Build history of the part. All positions in model axes, mm. A direction names the side the tool comes from. Round coordinates to 2 decimals unless told otherwise and drop trailing zeros. Write each loop counter-clockwise with the first axis right and the second up, starting at its lowest first coordinate (ties: lowest second). Pieces come first, ordered by that corner, then holes.
Item 1: Band-saw the part on A-A, the plane x = 0. Write the cut outline in (y, z).
Item 2: Wall check: probe 1 along X at (y, z) = (-1, 0); probe 2 along Z at (x, y) = (0, 2.1). Give the ranges that are in metal, low to high.
Item 3: Band-saw the part on D-D, the plane z = 2.25. Write the cut outline in (x, y), then the cut area to 3 significant figures.
Item 4: Drop a flat-ended pin along its axis: pin 1 Ø1 at (x, y) = (-2, -0.5) entering from -Z. Give the stop position or say it passes through.
Item 5: 3-axis set-ups, long thin cutter, end or side, ignore diameter. For faces 1 (the cylindrical face through (-6, -1, 0)), 2 (the cylindrical face through (3.233, 1.479, 1.341)): which of +Z, -Z, +X, -X, +Y, -Y reach the whole face in a straight line?
Item 6: Band-saw the part on C-C, the plane y = 2.1. Write the cut outline in (x, z).
Item 7: Band-saw the part on B-B, the plane z = 0.5. Write the cut outline in (x, y), then the cut area to 3 significant figures.
```python
from build123d import *

# Parameters (mm, degrees)
SKETCH_1_R      = 3.5
SKETCH_1_R_2    = 2
EXTRUDE_1_DEPTH = 3
SKETCH_1_3_R    = 6
SKETCH_1_3_R_2  = 3.5
SKETCH_1_3_R_3  = 2
EXTRUDE_2_DEPTH = 2


with BuildPart() as part:
    # Sketch 1 → Extrude 1 (new body)
    with BuildSketch(Plane(origin=(0, 0, 0), x_dir=(1, 0, 0), z_dir=(0, 1, 0))):
        Circle(SKETCH_1_R)
        Circle(SKETCH_1_R_2, mode=Mode.SUBTRACT)
    extrude(amount=EXTRUDE_1_DEPTH)

    # Sketch 1_3 → Extrude 2 (add)
    with BuildSketch(Plane(origin=(0, 0, 0), x_dir=(1, 0, 0), z_dir=(0, 1, 0))):
        Circle(SKETCH_1_3_R)
        Circle(SKETCH_1_3_R_2, mode=Mode.SUBTRACT)
        Circle(SKETCH_1_3_R_2)
        Circle(SKETCH_1_3_R_3, mode=Mode.SUBTRACT)
    extrude(amount=-EXTRUDE_2_DEPTH)


solid = part.part
```
Results:
1. outline: (-2, -6) - (0, -6) - (0, -3.5) - (3, -3.5) - (3, -2) - (-2, -2) - close; (-2, 2) - (3, 2) - (3, 3.5) - (0, 3.5) - (0, 6) - (-2, 6) - close
2. probe 1: x = -6 to -2, 2 to 6
2. probe 2: z = -3.5 to -2, 2 to 3.5
3. outline: (-5.56, -2) - (5.56, -2) - (5.56, 0) - (2.68, 0) - (2.68, 3) - (-2.68, 3) - (-2.68, 0) - (-5.56, 0) - close
3. area: 38.3 mm2
4. pin 1: stops at z = -5.81
5. face 1: +Y, -Y
5. face 2: +Y
6. outline: circle Ø7 at (0, 0); hole circle Ø4 at (0, 0)
7. outline: (-5.98, -2) - (-1.94, -2) - (-1.94, 3) - (-3.46, 3) - (-3.46, 0) - (-5.98, 0) - close; (1.94, -2) - (5.98, -2) - (5.98, 0) - (3.46, 0) - (3.46, 3) - (1.94, 3) - close
7. area: 25.3 mm2
